Could you check a few things on this drawing? It's one solid part, dimensions in mm from its lowest x, y, z. Coordinates: 2 decimals unless noted, no trailing zeros. Write each loop counter-clockwise with the first axis right and the second up, starting at its lowest first coordinate (ties: lowest second). Pieces come first, ordered by that corner, then holes. Notation, with made-up numbers: (-5.75, 53) - (46.25, 53) arc R19 cw to (46.25, 58) - close; hole circle Ø7 at (-29.75, -20). An arc over 180 degrees is marked (long way). Answer as a JSON object with one key per item and string values. Group by question number.
1) If we section it at C-C (z = 1.5): Write out the boundary of the cut face in (x, y), plus the area to 3 significant figures.
2) Please list where these lines run through material, in increasing order: line 1 along X through (y, z) = (16, 11); line 2 along Z through (x, y) = (13.75, 7); line 3 along X through (y, z) = (11, 3.5).
3) If we section it at A-A (y = 20.5): Write out the boundary of the cut face in (x, z).
4) Will these pins go through, and if not, where does the flat tip stop? pin 1 Ø1.6 at (x, y) = (29, 14) entering from -Z; pin 2 Ø1.9 at (y, z) = (15, 2) entering from +X; pin 3 Ø10 at (x, y) = (14.5, 12.5) entering from +Z.
5) We'd pull the mould along X, two halves only. Please class the marked faces 1, 2, 3 and 4: released by +X, released by -X, zero draft, split by the parting line, or undercut.
6) If we section it at B-B (x = 10.5): Write out the boundary of the cut face in (y, z).
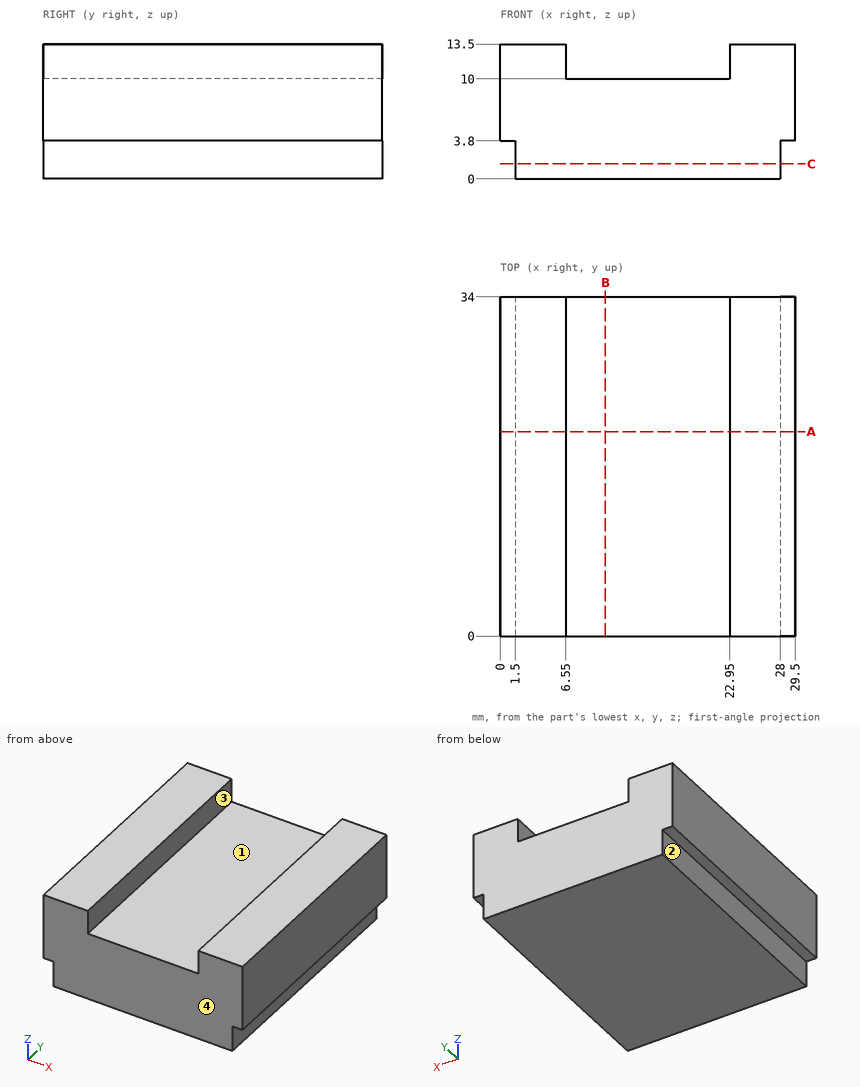
Here are the results:
{
 "1": {"outline": "(1.5, 0) - (28, 0) - (28, 34) - (1.5, 34) - close", "area": "901 mm²"},
 "2": {"line 1": "x = 0 to 6.55, 22.95 to 29.5", "line 2": "z = 0 to 10", "line 3": "x = 1.5 to 28"},
 "3": {"outline": "(0, 3.8) - (1.5, 3.8) - (1.5, 0) - (28, 0) - (28, 3.8) - (29.5, 3.8) - (29.5, 13.5) - (22.95, 13.5) - (22.95, 10) - (6.55, 10) - (6.55, 13.5) - (0, 13.5) - close"},
 "4": {"pin 1": "stops at z = 3.8", "pin 2": "stops at x = 28", "pin 3": "stops at z = 10"},
 "5": {"face 1": "undercut", "face 2": "released by -X", "face 3": "undercut", "face 4": "zero draft"},
 "6": {"outline": "(0, 0) - (34, 0) - (34, 10) - (0, 10) - close"}
}
